Design review of the part shown in the three views and the two pictorial views. Dimensions are in mm from the part's minimum x, y and z. A direction names the side the tool comes from. Give positions to 0.01 mm unless a question says otherwise; leave off trailing zeros. Write each loop counter-clockwise with the first axis right and the second up, starting at its lowest first coordinate (ties: lowest second). Pieces come first, ordered by that corner, then holes. Notation, with made-up numbers: M 24,-20 L 45,-20 A10 cw 45,-7 Z; hole C -37.75,84.25 d2. An arc over 180 degrees is marked long. Use one line per item in the form item = value. Start each with the question number.
Q1. For probe 1 along Y at (x, z) = (13.35, 5.25); probe 2 along Y at (x, z) = (13.75, 5.25) (1 decimal); probe 3 along Z at (x, y) = (20.75, 17.25), list the stretches that pass through material, from the lowest coordinate up. Write a range as [from, to].
Q2. Consider section C-C on y = 17. Write out the cut boundary in (x, z), and give its area (3 significant figures).
Q3. Consider section A-A on z = 4. Write out the cut boundary in (x, y).
Q4. Clearance check with flat-ended pins moving along their axes: pin 1 Ø2.5 at (x, y) = (13.35, 22.8) entering from +Z; pin 2 Ø1.5 at (x, z) = (17.5, 4) entering from -Y; pin 3 Ø3.5 at (x, y) = (2.895, 2.775) entering from +Z; pin 4 Ø2.5 at (x, y) = (23.805, 2.775) entering from +Z. State where each tip first meets the part, or that it passes through.
Q5. Consider section B-B on x = 19.75. Write out the cut boundary in (y, z).
Q6. Tool access review of the marked faces 1, 2, 3, 4 and 5: name each direction out of +Z, -Z, +X, -X, +Y, -Y from which nothing blocks a thin tool from reaching the whole face with its end or side.
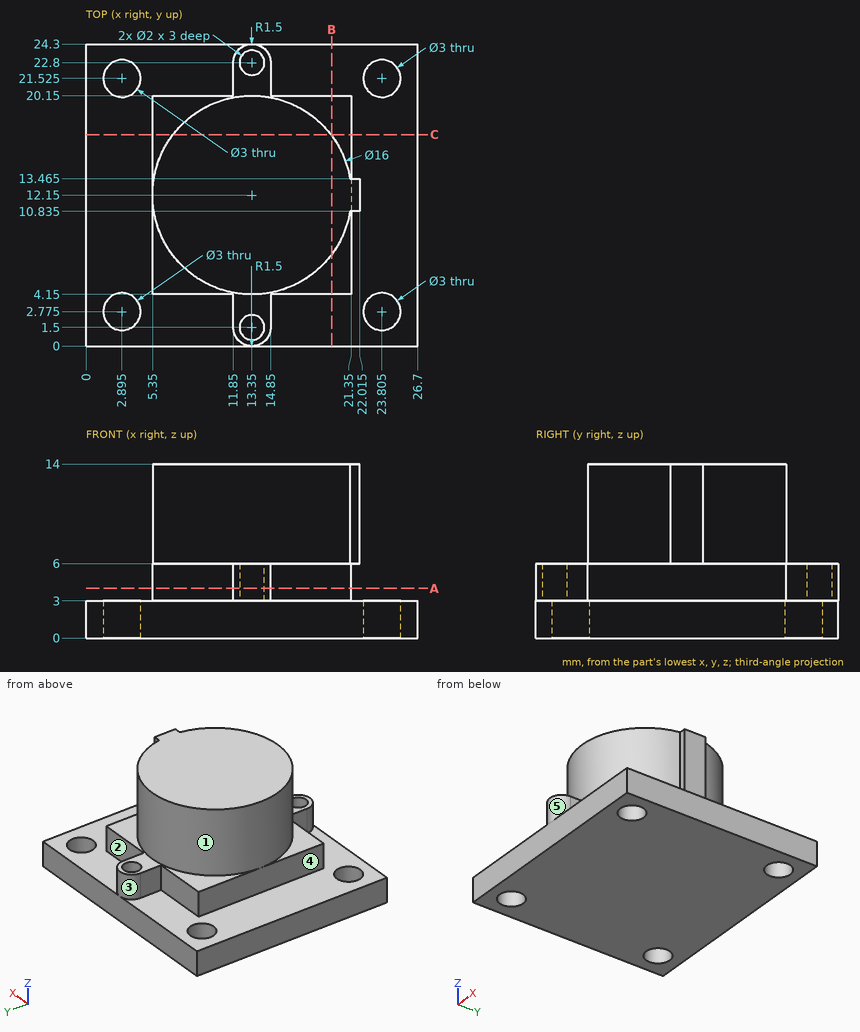
Working result:
q1.probe_1 = [0, 0.5], [2.5, 21.8], [23.8, 24.3]
q1.probe_2 = [0.1, 0.6], [2.4, 21.9], [23.7, 24.2]
q1.probe_3 = [0, 6]
q2.outline = M 0,0 L 26.7,0 L 26.7,3 L 21.35,3 L 21.35,6 L 19.71,6 L 19.71,14 L 6.99,14 L 6.99,6 L 5.35,6 L 5.35,3 L 0,3 Z
q2.area = 230 mm²
q3.outline = M 5.35,4.15 L 11.85,4.15 L 11.85,1.5 A1.5 ccw 14.85,1.5 L 14.85,4.15 L 21.35,4.15 L 21.35,20.15 L 14.85,20.15 L 14.85,22.8 A1.5 ccw 11.85,22.8 L 11.85,20.15 L 5.35,20.15 Z; hole C 13.35,1.5 d2; hole C 13.35,22.8 d2
q4.pin_1 = 6
q4.pin_2 = 4.15
q4.pin_3 = 3
q4.pin_4 = through
q5.outline = M 0,0 L 24.3,0 L 24.3,3 L 20.15,3 L 20.15,6 L 16.95,6 L 16.95,14 L 7.35,14 L 7.35,6 L 4.15,6 L 4.15,3 L 0,3 Z
q6.face_1 = +Z
q6.face_2 = +Z, +X, +Y
q6.face_3 = +Z, +Y
q6.face_4 = +Z, -X, +Y, -Y
q6.face_5 = +Z, -Y
